Here's how the part is built. I have some questions about the finished solid (model axes, mm). Coordinates: 2 decimals unless noted, no trailing zeros. Loops run counter-clockwise (first coordinate to the right, second up) from the corner with the lowest first, then second, coordinate; pieces in that order, holes last. Notation, with made-up numbers: M 89.25,35.25 L 140.25,35.25 A27 cw 140.25,60.25 Z; hole C 76.25,23.25 d2. An arc over 180 degrees is marked long. Use CSV: the item, a comma, the result in double quotes. Start each with the question number.
Q1. For pin 1 Ø6 at (y, z) = (46, 32) entering from -X; pin 2 Ø2 at (x, y) = (89.5, 49) entering from -Z; pin 3 Ø4 at (x, z) = (89.5, 39) entering from -Y; pin 4 Ø1 at (x, z) = (85, 22) entering from -Y, each with a flat end and sliding along its axis, tell me the tip position at first contact or that it passes through.
Q2. Please list where these lines run through material, in increasing order: probe 1 along Z at (x, y) = (85.75, 51.5); probe 2 along Z at (x, y) = (88.5, 50); probe 3 along X at (y, z) = (49.5, 67.5). Write a range as [from, to].
Q3. If we section it at A-A (z = 11): Please give me the cut outline in (x, y), and give its area (3 significant figures).
from build123d import *

# Parameters (mm, degrees)
EXTRUDE_2_DEPTH     = 75
SKETCH_5_R          = 1.5
CUT_EXTRUDE_1_DEPTH = 75
SKETCH_7_R          = 3
CUT_EXTRUDE_2_DEPTH = 3
CUT_EXTRUDE_3_DEPTH = 5


with BuildPart() as part:
    # Model → 凸台-拉伸2 (new body)
    with BuildSketch(Plane.XY):
        Polygon((81.281714853, 50.079307879), (85.170802149, 53.968395176), (91.53476318, 47.604434145), (87.645675883, 43.715346849), align=None)
    extrude(amount=EXTRUDE_2_DEPTH)

    # 草图5 → 切除-拉伸1 (cut)
    with BuildSketch(Plane(origin=(69.569598662, 69.569598663, 0), x_dir=(0, 0, -1), z_dir=(0.7071067811850318, 0.7071067811880632, 0))):
        with Locations(Location((-65, -26.56343356, 0), (0, 0, 90))):
            Circle(SKETCH_5_R)
        with Locations(Location((-45, -26.56343356, 0), (0, 0, 90))):
            Circle(SKETCH_5_R)
        with Locations(Location((-25, -26.56343356, 0), (0, 0, 90))):
            Circle(SKETCH_5_R)
        with Locations(Location((-5, -26.56343356, 0), (0, 0, 90))):
            Circle(SKETCH_5_R)
    extrude(amount=-CUT_EXTRUDE_1_DEPTH, mode=Mode.SUBTRACT)

    # 草图7 → 切除-拉伸2 (cut)
    with BuildSketch(Plane(origin=(69.569598662, 69.569598663, 0), x_dir=(0, 0, -1), z_dir=(0.7071067811850318, 0.7071067811880632, 0))):
        with Locations(Location((-5, -26.56343356, 0), (0, 0, 90))):
            Circle(SKETCH_7_R)
        with Locations(Location((-25, -26.56343356, 0), (0, 0, 90))):
            Circle(SKETCH_7_R)
        with Locations(Location((-45, -26.56343356, 0), (0, 0, 90))):
            Circle(SKETCH_7_R)
        with Locations(Location((-65, -26.56343356, 0), (0, 0, 90))):
            Circle(SKETCH_7_R)
    extrude(amount=-CUT_EXTRUDE_2_DEPTH, mode=Mode.SUBTRACT)

    # 草图8 → 切除-拉伸3 (cut)
    with BuildSketch(Plane.XY.offset(75)):
        Polygon((87.645675883, 43.715346849), (91.53476318, 47.604434145), (85.134022188, 54.005175138), (81.244934891, 50.116087842), align=None)
    extrude(amount=-CUT_EXTRUDE_3_DEPTH, mode=Mode.SUBTRACT)


solid = part.part
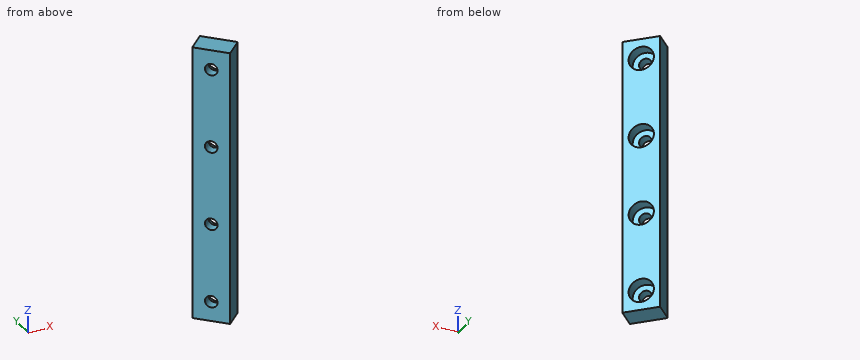
Results below:
1,pin 1,"x = 82.36"
1,pin 2,"z = 0"
1,pin 3,"y = 43.72"
1,pin 4,"y = 45.86"
2,probe 1,"[0, 3.13], [6.87, 23.13], [26.87, 43.13], [46.87, 63.13], [66.87, 70]"
2,probe 2,"[0, 2.07], [7.93, 22.07], [27.93, 42.07], [47.93, 62.07], [67.93, 70]"
2,probe 3,"[81.86, 85.4], [89.41, 89.64]"
3,outline,"M 81.28,50.08 L 87.65,43.72 L 91.53,47.6 L 85.17,53.97 Z"
3,area,"49.5 mm^2"
